from build123d import *

# Parameters (mm, degrees)
F0_W     = 30
F0_H     = 15
F1_DEPTH = 2


with BuildPart() as f1:
    # F0 (on Top) → F1 (new body)
    with BuildSketch(Plane.XY):
        with Locations((-15, 7.5)):
            Rectangle(F0_W, F0_H)
        with BuildLine():
            add(Edge.make_bspline(
                [(-25.2514986596, 6.1214301728), (-25.723342297, 5.6079070142), (-26.6088355231, 5.6079070142)],
                knots=[0, 0, 0, 1, 1, 1], degree=2))
            add(Edge.make_bspline(
                [(-26.6088355231, 5.6079070142), (-27.0696694756, 5.6079070142), (-27.3354747247, 5.7400232326)],
                knots=[0, 0, 0, 1, 1, 1], degree=2))
            Line((-27.3354747247, 5.7400232326), (-27.3354747247, 6.4525071251))
            add(Edge.make_bspline(
                [(-27.3354747247, 6.4525071251), (-26.986310433, 6.3549927733), (-26.6088355231, 6.3549927733)],
                knots=[0, 0, 0, 1, 1, 1], degree=2))
            add(Edge.make_bspline(
                [(-26.6088355231, 6.3549927733), (-26.1212637645, 6.3549927733), (-25.8680410125, 6.6498950467)],
                knots=[0, 0, 0, 1, 1, 1], degree=2))
            add(Edge.make_bspline(
                [(-25.8680410125, 6.6498950467), (-25.6148182604, 6.94479732), (-25.6148182604, 7.5)],
                knots=[0, 0, 0, 1, 1, 1], degree=2))
            Line((-25.6148182604, 7.5), (-25.6148182604, 14.6861785971))
            Line((-25.6148182604, 14.6861785971), (-24.7796550223, 14.6861785971))
            Line((-24.7796550223, 14.6861785971), (-24.7796550223, 7.5692037335))
            add(Edge.make_bspline(
                [(-24.7796550223, 7.5692037335), (-24.7796550223, 6.6349533315), (-25.2514986596, 6.1214301728)],
                knots=[0, 0, 0, 1, 1, 1], degree=2))
        make_face(mode=Mode.SUBTRACT)
        with BuildLine():
            Line((-19.0782110708, 7.5), (-19.6837437387, 7.5))
            Line((-19.6837437387, 7.5), (-19.8457433876, 8.2675323168))
            Line((-19.8457433876, 8.2675323168), (-19.8850636907, 8.2675323168))
            add(Edge.make_bspline(
                [(-19.8850636907, 8.2675323168), (-20.2877035946, 7.7610868127), (-20.6879842802, 7.5809998244)],
                knots=[0, 0, 0, 1, 1, 1], degree=2))
            add(Edge.make_bspline(
                [(-20.6879842802, 7.5809998244), (-21.0882649659, 7.4009128362), (-21.6890791975, 7.4009128362)],
                knots=[0, 0, 0, 1, 1, 1], degree=2))
            add(Edge.make_bspline(
                [(-21.6890791975, 7.4009128362), (-22.4896405689, 7.4009128362), (-22.9441832729, 7.8145624249)],
                knots=[0, 0, 0, 1, 1, 1], degree=2))
            add(Edge.make_bspline(
                [(-22.9441832729, 7.8145624249), (-23.3987259769, 8.2282120137), (-23.3987259769, 8.9894530819)],
                knots=[0, 0, 0, 1, 1, 1], degree=2))
            add(Edge.make_bspline(
                [(-23.3987259769, 8.9894530819), (-23.3987259769, 10.6204592551), (-20.7894306623, 10.6990998613)],
                knots=[0, 0, 0, 1, 1, 1], degree=2))
            Line((-20.7894306623, 10.6990998613), (-19.8756268179, 10.7289832917))
            Line((-19.8756268179, 10.7289832917), (-19.8756268179, 11.0639922742))
            add(Edge.make_bspline(
                [(-19.8756268179, 11.0639922742), (-19.8756268179, 11.6978355604), (-20.1477233155, 11.9998154883)],
                knots=[0, 0, 0, 1, 1, 1], degree=2))
            add(Edge.make_bspline(
                [(-20.1477233155, 11.9998154883), (-20.419819813, 12.3017954162), (-21.0206340446, 12.3017954162)],
                knots=[0, 0, 0, 1, 1, 1], degree=2))
            add(Edge.make_bspline(
                [(-21.0206340446, 12.3017954162), (-21.6937976339, 12.3017954162), (-22.5431161812, 11.8897186396)],
                knots=[0, 0, 0, 1, 1, 1], degree=2))
            Line((-22.5431161812, 11.8897186396), (-22.7947661211, 12.5141250531))
            add(Edge.make_bspline(
                [(-22.7947661211, 12.5141250531), (-22.3968446536, 12.7296003141), (-21.922641798, 12.8522796598)],
                knots=[0, 0, 0, 1, 1, 1], degree=2))
            add(Edge.make_bspline(
                [(-21.922641798, 12.8522796598), (-21.4484389425, 12.9749590056), (-20.9703040566, 12.9749590056)],
                knots=[0, 0, 0, 1, 1, 1], degree=2))
            add(Edge.make_bspline(
                [(-20.9703040566, 12.9749590056), (-20.0077430364, 12.9749590056), (-19.5429770536, 12.5479405137)],
                knots=[0, 0, 0, 1, 1, 1], degree=2))
            add(Edge.make_bspline(
                [(-19.5429770536, 12.5479405137), (-19.0782110708, 12.1209220219), (-19.0782110708, 11.1772347472)],
                knots=[0, 0, 0, 1, 1, 1], degree=2))
            Line((-19.0782110708, 11.1772347472), (-19.0782110708, 7.5))
        make_face(mode=Mode.SUBTRACT)
        with BuildLine():
            Line((-12.8954866092, 7.5), (-13.7117761018, 7.5))
            Line((-13.7117761018, 7.5), (-13.7117761018, 10.985351668))
            add(Edge.make_bspline(
                [(-13.7117761018, 10.985351668), (-13.7117761018, 11.6427871361), (-14.0113968115, 11.9675728398)],
                knots=[0, 0, 0, 1, 1, 1], degree=2))
            add(Edge.make_bspline(
                [(-14.0113968115, 11.9675728398), (-14.3110175213, 12.2923585435), (-14.951152056, 12.2923585435)],
                knots=[0, 0, 0, 1, 1, 1], degree=2))
            add(Edge.make_bspline(
                [(-14.951152056, 12.2923585435), (-15.7957521668, 12.2923585435), (-16.188955198, 11.8354566213)],
                knots=[0, 0, 0, 1, 1, 1], degree=2))
            add(Edge.make_bspline(
                [(-16.188955198, 11.8354566213), (-16.5821582291, 11.3785546991), (-16.5821582291, 10.3263433878)],
                knots=[0, 0, 0, 1, 1, 1], degree=2))
            Line((-16.5821582291, 10.3263433878), (-16.5821582291, 7.5))
            Line((-16.5821582291, 7.5), (-17.3984477218, 7.5))
            Line((-17.3984477218, 7.5), (-17.3984477218, 12.8868815266))
            Line((-17.3984477218, 12.8868815266), (-16.7347210052, 12.8868815266))
            Line((-16.7347210052, 12.8868815266), (-16.6026047867, 12.1492326402))
            Line((-16.6026047867, 12.1492326402), (-16.5632844836, 12.1492326402))
            add(Edge.make_bspline(
                [(-16.5632844836, 12.1492326402), (-16.3116345437, 12.5471541077), (-15.8594510579, 12.7665613991)],
                knots=[0, 0, 0, 1, 1, 1], degree=2))
            add(Edge.make_bspline(
                [(-15.8594510579, 12.7665613991), (-15.4072675721, 12.9859686904), (-14.8520648921, 12.9859686904)],
                knots=[0, 0, 0, 1, 1, 1], degree=2))
            add(Edge.make_bspline(
                [(-14.8520648921, 12.9859686904), (-13.878494187, 12.9859686904), (-13.3869903981, 12.5164842712)],
                knots=[0, 0, 0, 1, 1, 1], degree=2))
            add(Edge.make_bspline(
                [(-13.3869903981, 12.5164842712), (-12.8954866092, 12.0469998521), (-12.8954866092, 11.0136622862)],
                knots=[0, 0, 0, 1, 1, 1], degree=2))
            Line((-12.8954866092, 11.0136622862), (-12.8954866092, 7.5))
        make_face(mode=Mode.SUBTRACT)
        with BuildLine():
            Line((-6.7174805839, 7.5), (-7.5337700766, 7.5))
            Line((-7.5337700766, 7.5), (-7.5337700766, 10.985351668))
            add(Edge.make_bspline(
                [(-7.5337700766, 10.985351668), (-7.5337700766, 11.6427871361), (-7.8333907863, 11.9675728398)],
                knots=[0, 0, 0, 1, 1, 1], degree=2))
            add(Edge.make_bspline(
                [(-7.8333907863, 11.9675728398), (-8.133011496, 12.2923585435), (-8.7731460307, 12.2923585435)],
                knots=[0, 0, 0, 1, 1, 1], degree=2))
            add(Edge.make_bspline(
                [(-8.7731460307, 12.2923585435), (-9.6177461416, 12.2923585435), (-10.0109491728, 11.8354566213)],
                knots=[0, 0, 0, 1, 1, 1], degree=2))
            add(Edge.make_bspline(
                [(-10.0109491728, 11.8354566213), (-10.4041522039, 11.3785546991), (-10.4041522039, 10.3263433878)],
                knots=[0, 0, 0, 1, 1, 1], degree=2))
            Line((-10.4041522039, 10.3263433878), (-10.4041522039, 7.5))
            Line((-10.4041522039, 7.5), (-11.2204416965, 7.5))
            Line((-11.2204416965, 7.5), (-11.2204416965, 12.8868815266))
            Line((-11.2204416965, 12.8868815266), (-10.55671498, 12.8868815266))
            Line((-10.55671498, 12.8868815266), (-10.4245987615, 12.1492326402))
            Line((-10.4245987615, 12.1492326402), (-10.3852784584, 12.1492326402))
            add(Edge.make_bspline(
                [(-10.3852784584, 12.1492326402), (-10.1336285185, 12.5471541077), (-9.6814450327, 12.7665613991)],
                knots=[0, 0, 0, 1, 1, 1], degree=2))
            add(Edge.make_bspline(
                [(-9.6814450327, 12.7665613991), (-9.2292615469, 12.9859686904), (-8.6740588669, 12.9859686904)],
                knots=[0, 0, 0, 1, 1, 1], degree=2))
            add(Edge.make_bspline(
                [(-8.6740588669, 12.9859686904), (-7.7004881618, 12.9859686904), (-7.2089843729, 12.5164842712)],
                knots=[0, 0, 0, 1, 1, 1], degree=2))
            add(Edge.make_bspline(
                [(-7.2089843729, 12.5164842712), (-6.7174805839, 12.0469998521), (-6.7174805839, 11.0136622862)],
                knots=[0, 0, 0, 1, 1, 1], degree=2))
            Line((-6.7174805839, 11.0136622862), (-6.7174805839, 7.5))
        make_face(mode=Mode.SUBTRACT)
        with BuildLine():
            add(Edge.make_bspline(
                [(-1.8354717493, 7.4826990666), (-2.2208107199, 7.4009128362), (-2.7665765271, 7.4009128362)],
                knots=[0, 0, 0, 1, 1, 1], degree=2))
            add(Edge.make_bspline(
                [(-2.7665765271, 7.4009128362), (-3.9603409296, 7.4009128362), (-4.6515918584, 8.1291248498)],
                knots=[0, 0, 0, 1, 1, 1], degree=2))
            add(Edge.make_bspline(
                [(-4.6515918584, 8.1291248498), (-5.3428427871, 8.8573368635), (-5.3428427871, 10.1486156177)],
                knots=[0, 0, 0, 1, 1, 1], degree=2))
            add(Edge.make_bspline(
                [(-5.3428427871, 10.1486156177), (-5.3428427871, 11.452476869), (-4.7011354403, 12.2192227797)],
                knots=[0, 0, 0, 1, 1, 1], degree=2))
            add(Edge.make_bspline(
                [(-4.7011354403, 12.2192227797), (-4.0594280935, 12.9859686904), (-2.9773333518, 12.9859686904)],
                knots=[0, 0, 0, 1, 1, 1], degree=2))
            add(Edge.make_bspline(
                [(-2.9773333518, 12.9859686904), (-1.9660151557, 12.9859686904), (-1.376210609, 12.3198827557)],
                knots=[0, 0, 0, 1, 1, 1], degree=2))
            add(Edge.make_bspline(
                [(-1.376210609, 12.3198827557), (-0.7864060623, 11.6537968209), (-0.7864060623, 10.5622652065)],
                knots=[0, 0, 0, 1, 1, 1], degree=2))
            Line((-0.7864060623, 10.5622652065), (-0.7864060623, 10.0463828296))
            Line((-0.7864060623, 10.0463828296), (-4.4966698641, 10.0463828296))
            add(Edge.make_bspline(
                [(-4.4966698641, 10.0463828296), (-4.4715048701, 9.0979771185), (-4.0169621661, 8.6064733296)],
                knots=[0, 0, 0, 1, 1, 1], degree=2))
            add(Edge.make_bspline(
                [(-4.0169621661, 8.6064733296), (-3.5624194621, 8.1149695407), (-2.7366930967, 8.1149695407)],
                knots=[0, 0, 0, 1, 1, 1], degree=2))
            add(Edge.make_bspline(
                [(-2.7366930967, 8.1149695407), (-1.8669279918, 8.1149695407), (-1.0176094446, 8.4782891415)],
                knots=[0, 0, 0, 1, 1, 1], degree=2))
            Line((-1.0176094446, 8.4782891415), (-1.0176094446, 7.7500771278))
            add(Edge.make_bspline(
                [(-1.0176094446, 7.7500771278), (-1.4501327788, 7.5644852971), (-1.8354717493, 7.4826990666)],
                knots=[0, 0, 0, 1, 1, 1], degree=2))
        make_face(mode=Mode.SUBTRACT)
    extrude(amount=-F1_DEPTH)


solid = f1.part
CAD build for the part. Positions are in the model's coordinates, mm. A direction names the side the tool comes from. Round coordinates to 2 decimals unless told otherwise and drop trailing zeros. One line per question, with ' | ' between items. Start each with the question number.
Item 1: Wall check: line 1 (Y direction, x = -26.5, z = -1.45); line 2 (Y direction, x = -2.5, z = -0.45); line 3 (Y direction, x = -21, z = -1.35). Give the ranges that are in metal, low to high.
Item 2: Cut at A-A, the plane z = -1.3. State how many separate pieces and enclosed holes the cut face has, plus the area to 3 significant figures.
Item 3: Two-plate mould, pull along X, no slides. Class faces 1 (the flat face through (-15, 0, -1)), 2 (the flat face through (0, 7, -1)), 3 (the flat face through (-25.615, 11, -1)), 4 (the flat face through (-30, 7, -1)): pulls with the +X half, pulls with the -X half, needs draft (parallel to the pull), parting line crosses it, or undercut.
Item 4: Which spindle directions (+Z, -Z, +X, -X, +Y, -Y) get a long thin tool onto all of the face, cutting with end or side? Do faces 5 (the flat face through (-10.404, 9, -1)), 6 (the flat face through (-15, 8, -2)). Say none if no direction does.
Responses:
1) line 1: y = 0 to 5.61, 6.36 to 15 | line 2: y = 0 to 7.41, 8.12 to 10.05, 12.94 to 15 | line 3: y = 0 to 7.48, 10.69 to 12.3, 12.97 to 15
2) separate pieces: 1 | enclosed holes: 5 | area: 390 mm²
3) face 1: needs draft | face 2: pulls with the +X half | face 3: undercut | face 4: pulls with the -X half
4) face 5: +Z, -Z | face 6: -Z, +X, -X, +Y, -Y
